For this review, take the finished solid that the model builds, in its own axes (mm). A direction names the side the tool comes from. Give positions to 0.01 mm unless a question says otherwise; leave off trailing zeros. Write each loop counter-clockwise with the first axis right and the second up, starting at its lowest first coordinate (ties: lowest second). Pieces come first, ordered by that corner, then holes.
1) We need section C-C on z = 16.5. Give the boundary of the cut face in (x, y).
2) We need section A-A on y = 29.5. Give the boundary of the cut face in (x, z).
3) Machinability: for faces 1 (the face through (-18.5, 27.6, -12.3)), 2 (the face through (0, 28, 28)), 3 (the face through (-20, 28, -12)), 4 (the face through (-13.25, 10.06, 26.52)), which of the approach directions +Z, -Z, +X, -X, +Y, -Y give a long, thin tool a straight path to every point of the face, cutting with its end or side? Answer none if there is none.
4) Wall thickness on line 1 along Z through (x, y) = (-19, 8); line 2 along Z through (x, y) = (-20, 48); line 3 along X through (y, z) = (50, 15.5): over which ranges is each line inside the solid? List them lowest first.
5) We need section B-B on x = 5. Give the boundary of the cut face in (y, z), and give its area (3 significant figures).
6) We need section D-D on x = -14.5. Give the boundary of the cut face in (y, z).
7) For P1, Ø2, axis at y = 48, z = -15.85, coming from the +X side; P2, Ø17, axis at x = -3.5, y = 25.5, coming from the -Z side; P3, Ø5.5, axis at y = 48, z = 12.15, coming from the -X side; P4, Ø4, axis at y = 8, z = -15.85, coming from the -X side, all flat-tipped, find the tip position at first contact; note any pin that passes through.
8) Draft analysis for pull direction Y (two halves, no side actions). For faces 5 (the face through (-20, 28, -25)), 6 (the face through (-20, 9, -2)), 7 (the face through (-19.68, 46.61, -14.96)), state which applies: pulls with the +Y half, pulls with the -Y half, needs draft (parallel to the pull), parting line crosses it, or undercut.
from build123d import *

# Parameters (mm, degrees)
EXTRUDE_1_DEPTH              = 56
FILLET_1_R                   = 3
FILLET_2_R                   = 0.5
CUT_EXTRUDE_1_REACH          = 82.045
CUT_EXTRUDE_2_REACH          = 76.297
HOLE_WIZARD_M4_1_D           = 3.3
HOLE_WIZARD_M4_1_CSINK_D     = 4.5
HOLE_WIZARD_M4_1_CSINK_ANGLE = 90


with BuildPart() as part:
    # 草图1 → 拉伸-薄壁1 (new body)
    with BuildSketch(Plane(origin=(0, 0, 0), x_dir=(1, 0, 0), z_dir=(0, 1, 0))):
        Polygon((-18.5, 25), (-18.5, -25), (18.5, -25), (18.5, -28), (-21.5, -28), (-21.5, 25), align=None)
    extrude(amount=EXTRUDE_1_DEPTH)

    # 圆角1
    fillet_1_edges = [part.edges().sort_by_distance(p)[0] for p in [
        (-21.5, 28, 28),
        (-18.5, 28, 25),
    ]]
    fillet(fillet_1_edges, radius=FILLET_1_R)

    # 圆角2
    fillet_2_edges = [part.edges().sort_by_distance(p)[0] for p in [
        (0, 0, 28),
        (18.5, 0, 26.5),
        (1.5, 0, 25),
        (-18.5, 0, -1.5),
        (-20, 0, -25),
        (-21.5, 0, 0),
        (18.5, 56, 26.5),
        (1.5, 56, 25),
        (-18.5, 56, -1.5),
        (-20, 56, -25),
        (-21.5, 56, 0),
        (0, 56, 28),
        (-20.621320344, 0, 27.121320344),
        (-20.621320344, 56, 27.121320344),
    ]]
    fillet(fillet_2_edges, radius=FILLET_2_R)

    # 草图2 → 切除-拉伸1 (cut, up to next)
    with BuildSketch(Plane.XY.offset(28), mode=Mode.PRIVATE) as cut_extrude_1_sk1:
        with BuildLine():
            Line((-10.5, 48.75), (9.5, 48.75))
            ThreePointArc((9.5, 48.75), (12.25, 46), (9.5, 43.25))
            Line((9.5, 43.25), (-10.5, 43.25))
            ThreePointArc((-10.5, 43.25), (-13.25, 46), (-10.5, 48.75))
        make_face()
    cut_extrude_1_tool1 = extrude(cut_extrude_1_sk1.sketch, amount=-CUT_EXTRUDE_1_REACH, mode=Mode.PRIVATE) & part.part
    # 草图2 → 切除-拉伸1 (cut, up to next)
    with BuildSketch(Plane.XY.offset(28), mode=Mode.PRIVATE) as cut_extrude_1_sk2:
        with BuildLine():
            Line((-10.5, 7.25), (9.5, 7.25))
            ThreePointArc((9.5, 7.25), (12.25, 10), (9.5, 12.75))
            Line((9.5, 12.75), (-10.5, 12.75))
            ThreePointArc((-10.5, 12.75), (-13.25, 10), (-10.5, 7.25))
        make_face()
    cut_extrude_1_tool2 = extrude(cut_extrude_1_sk2.sketch, amount=-CUT_EXTRUDE_1_REACH, mode=Mode.PRIVATE) & part.part
    add(cut_extrude_1_tool1.solids().sort_by_distance((-0.5, 46, 28))[0], mode=Mode.SUBTRACT)
    add(cut_extrude_1_tool2.solids().sort_by_distance((-0.5, 10, 28))[0], mode=Mode.SUBTRACT)

    # 草图3 → 切除-拉伸2 (cut, up to next)
    with BuildSketch(Plane.ZY.offset(21.5), mode=Mode.PRIVATE) as cut_extrude_2_sk1:
        with BuildLine():
            Line((-12, 19), (-12, 37))
            ThreePointArc((-12, 37), (-2, 47), (8, 37))
            Line((8, 37), (8, 19))
            ThreePointArc((8, 19), (-2, 9), (-12, 19))
        make_face()
    cut_extrude_2_tool1 = extrude(cut_extrude_2_sk1.sketch, amount=-CUT_EXTRUDE_2_REACH, mode=Mode.PRIVATE) & part.part
    add(cut_extrude_2_tool1.solids().sort_by_distance((-21.5, 28, -2))[0], mode=Mode.SUBTRACT)

    # M4 螺纹孔1 (through all)
    with Locations(Plane(origin=(-21.5, 8, -15.849623113), x_dir=(0, 0, -1), z_dir=(-1, 0, 0))):
        with Locations((0, 0), (-14, -20), (0, -40), (-28, -40), (-28, 0)):
            CounterSinkHole(HOLE_WIZARD_M4_1_D / 2, HOLE_WIZARD_M4_1_CSINK_D / 2, counter_sink_angle=HOLE_WIZARD_M4_1_CSINK_ANGLE)


solid = part.part
Results list:
1. outline: (-21.5, 0.5) arc R0.5 ccw to (-21, 0) - (-19, 0) arc R0.5 ccw to (-18.5, 0.5) - (-18.5, 55.5) arc R0.5 ccw to (-19, 56) - (-21, 56) arc R0.5 ccw to (-21.5, 55.5) - close
2. outline: (-21.5, -25) - (-18.5, -25) - (-18.5, -12) - (-21.5, -12) - close; (-21.5, 8) - (-18.5, 8) - (-18.5, 22) arc R3 cw to (-15.5, 25) - (18.5, 25) - (18.5, 28) - (-18.5, 28) arc R3 ccw to (-21.5, 25) - close
3. face 1: -Z, +X, +Y, -Y
3. face 2: +Z, +X, -X, +Y, -Y
3. face 3: +X, -X
3. face 4: +Z, -Z
4. line 1: z = -25 to -17.5, -14.2 to 10.5, 13.8 to 27.96
4. line 2: z = -25 to -17.5, -14.2 to 10.5, 13.8 to 27.6
4. line 3: x = -21.5 to -18.5
5. outline: (0, 25.5) arc R0.5 ccw to (0.5, 25) - (7.25, 25) - (7.25, 28) - (0.5, 28) arc R0.5 ccw to (0, 27.5) - close; (12.75, 25) - (43.25, 25) - (43.25, 28) - (12.75, 28) - close; (48.75, 25) - (55.5, 25) arc R0.5 ccw to (56, 25.5) - (56, 27.5) arc R0.5 ccw to (55.5, 28) - (48.75, 28) - close
5. area: 135 mm2
6. outline: (0, 25.5) arc R0.5 ccw to (0.5, 25) - (55.5, 25) arc R0.5 ccw to (56, 25.5) - (56, 27.5) arc R0.5 ccw to (55.5, 28) - (0.5, 28) arc R0.5 ccw to (0, 27.5) - close
7. P1: passes through
7. P2: stops at z = 25
7. P3: stops at x = -21.5
7. P4: stops at x = -21.25
8. face 5: needs draft
8. face 6: undercut
8. face 7: undercut
